Could you check a few things on this drawing? It's one solid part, dimensions in mm from its lowest x, y, z. A direction names the side the tool comes from. Give positions to 0.01 mm unless a question says otherwise; leave off trailing zeros. Order: outer loops, then holes, each group sorted by start corner. A loop starts at its lowest first (then second) coordinate and runs counter-clockwise, first axis right, second up. Notation, with made-up numbers: (80.25, -14) -> (114.25, -14) arc R14 ccw to (114.25, -4) -> close; hole circle Ø8 at (19, -32.5). An arc over 180 degrees is marked (long way). Use one line per item in the form item = value. Start each with the question number.
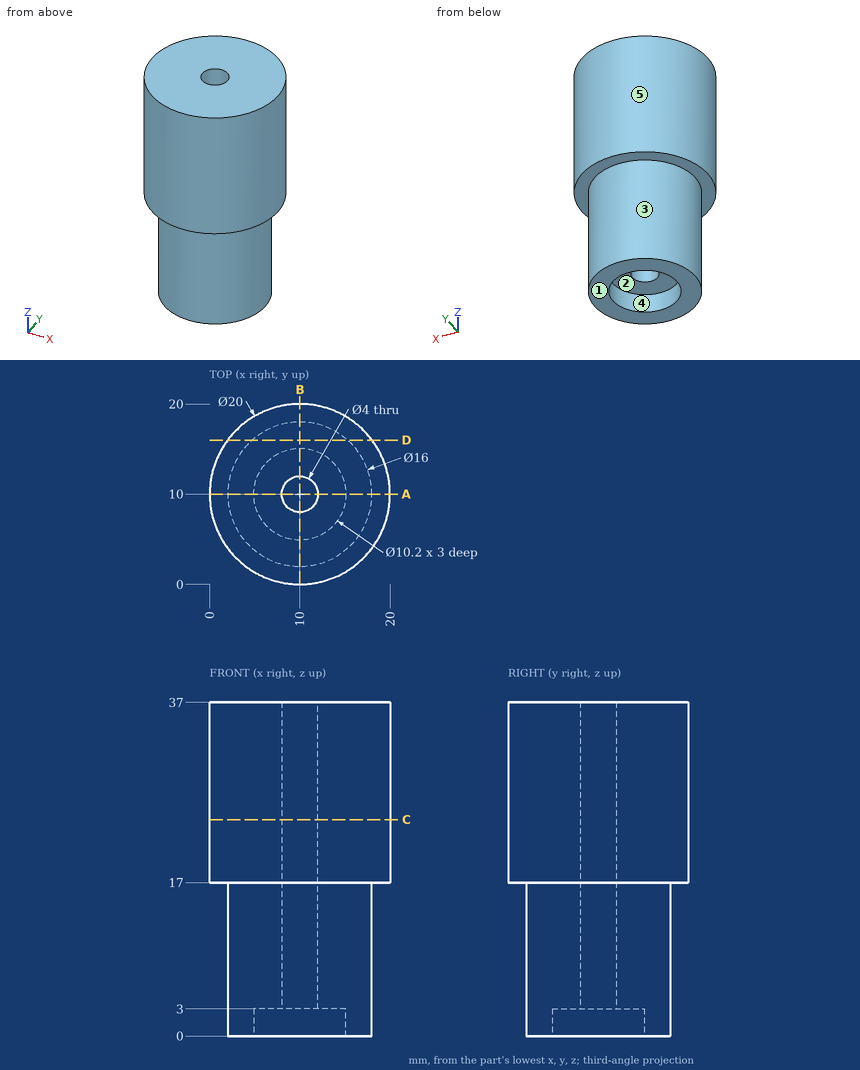
(1) Imagine slicing it at D-D (y = 16). Write out the boundary of the cut face in (x, z), plus the area to 3 significant figures.
(2) Imagine slicing it at A-A (y = 10). Write out the boundary of the cut face in (x, z), plus the area to 3 significant figures.
(3) I'm going to push flat-ended pins straight in: pin 1 Ø1 at (x, z) = (5, 23) entering from -Y; pin 2 Ø4 at (x, z) = (11, 11.5) entering from -Y; pin 3 Ø8 at (x, y) = (10, 10) entering from -Z. Where does each tip first touch, or does it pass through?
(4) We'd pull the mould along X, two halves only. Please class the marked faces 1, 2 and 3: pulls with the +X half, pulls with the -X half, needs draft (parallel to the pull), parting line crosses it, or undercut.
(5) Please list where these lines run through material, in increasing order: probe 1 along X at (y, z) = (10, 23); probe 2 along Z at (x, y) = (17.25, 3.25); probe 3 along Z at (x, y) = (6.25, 11.25).
(6) Imagine slicing it at C-C (z = 24). Write out the boundary of the cut face in (x, y), plus the area to 3 significant figures.
(7) Which directions (+Z, -Z, +X, -X, +Y, -Y) give clear straight access to the entire face, cutting with the end or side of a thin tool? Please do the marked faces 4 and 5.
Calculated:
q1.outline = (2, 17) -> (4.71, 17) -> (4.71, 0) -> (15.29, 0) -> (15.29, 17) -> (18, 17) -> (18, 37) -> (2, 37) -> close
q1.area = 500 mm2
q2.outline = (0, 17) -> (2, 17) -> (2, 0) -> (4.9, 0) -> (4.9, 3) -> (8, 3) -> (8, 37) -> (0, 37) -> close; (12, 3) -> (15.1, 3) -> (15.1, 0) -> (18, 0) -> (18, 17) -> (20, 17) -> (20, 37) -> (12, 37) -> close
q2.area = 505 mm2
q3.pin_1 = 1.07
q3.pin_2 = 2
q3.pin_3 = 3
q4.face_1 = needs draft
q4.face_2 = undercut
q4.face_3 = parting line crosses it
q5.probe_1 = 0 to 8, 12 to 20
q5.probe_2 = 17 to 37
q5.probe_3 = 3 to 37
q6.outline = circle Ø20 at (10, 10); hole circle Ø4 at (10, 10)
q6.area = 302 mm2
q7.face_4 = -Z
q7.face_5 = +Z, -Z
